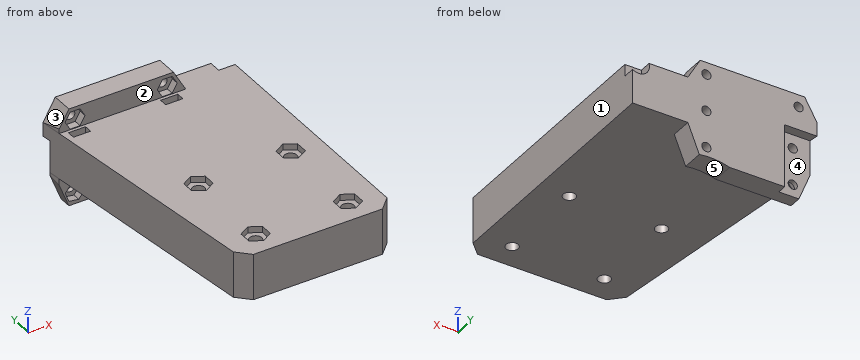
```python
from build123d import *

# Parameters (mm, degrees)
SKETCH1_W               = 50
SKETCH1_H               = 70
BOSS_EXTRUDE1_DEPTH     = 15
SKETCH3_R               = 2
CUT_EXTRUDE1_DEPTH      = 16
SKETCH4_W               = 50
SKETCH4_H               = 15
BOSS_EXTRUDE2_DEPTH     = 16
CHAMFER1_SIZE           = 4
BOSS_EXTRUDE3_DEPTH     = 15
SKETCH6_R               = 3.5
CUT_EXTRUDE2_DEPTH      = 4
SKETCH7_R               = 1.5
BOSS_EXTRUDE4_DEPTH     = 7
CUT_EXTRUDE3_DEPTH      = 8
CUT_EXTRUDE3_DEPTH_BACK = 26
SKETCH7_2_R             = 1.5
CUT_EXTRUDE4_DEPTH      = 20
SKETCH9_W               = 5.6
SKETCH9_H               = 2.6
CUT_EXTRUDE5_DEPTH      = 26
SKETCH10_W              = 10.5
SKETCH10_H              = 20.5
CUT_EXTRUDE6_DEPTH      = 3
CUT_EXTRUDE7_DEPTH      = 2.5
CUT_EXTRUDE8_DEPTH      = 2
SKETCH14_R              = 22
CUT_EXTRUDE9_DEPTH      = 87


with BuildPart() as part:
    # Sketch1 → Boss-Extrude1 (new body)
    with BuildSketch(Plane.XY):
        Rectangle(SKETCH1_W, SKETCH1_H)
    extrude(amount=BOSS_EXTRUDE1_DEPTH)

    # Sketch3 → Cut-Extrude1 (cut, through all)
    with BuildSketch(Plane.XY.offset(15)):
        with Locations((-15, 2.7)):
            Circle(SKETCH3_R)
        with Locations((15, 2.7)):
            Circle(SKETCH3_R)
        with Locations((-15, -26.7)):
            Circle(SKETCH3_R)
        with Locations((15, -26.7)):
            Circle(SKETCH3_R)
    extrude(amount=-CUT_EXTRUDE1_DEPTH, mode=Mode.SUBTRACT)

    # Sketch4 → Boss-Extrude2 (add)
    with BuildSketch(Plane(origin=(0, 35, 0), x_dir=(1, 0, 0), z_dir=(0, 1, 0))):
        with Locations((0, -7.5)):
            Rectangle(SKETCH4_W, SKETCH4_H)
    extrude(amount=BOSS_EXTRUDE2_DEPTH)

    # Chamfer1
    chamfer1_edges = [part.edges().sort_by_distance(p)[0] for p in [
        (25, -35, 7.5),
        (-25, -35, 7.5),
    ]]
    chamfer(chamfer1_edges, length=CHAMFER1_SIZE)

    # Sketch5 → Boss-Extrude3 (add)
    with BuildSketch(Plane.XY.offset(15)):
        Polygon((-25, 51), (-35, 51), (-25, -31), align=None)
    extrude(amount=-BOSS_EXTRUDE3_DEPTH)

    # Sketch6 → Cut-Extrude2 (cut)
    with BuildSketch(Plane(origin=(0, 51, 0), x_dir=(1, 0, 0), z_dir=(0, 1, 0))):
        with Locations((23, -14)):
            Circle(SKETCH6_R)
    extrude(amount=-CUT_EXTRUDE2_DEPTH, mode=Mode.SUBTRACT)

    # Sketch7 → Boss-Extrude4 (add)
    with BuildSketch(Plane(origin=(0, 51, 0), x_dir=(1, 0, 0), z_dir=(0, 1, 0))):
        with Locations((-29, -6)):
            Circle(SKETCH7_R)
        with Locations((1, -6)):
            Circle(SKETCH7_R)
        Polygon((-35, -15), (-31, -22), (3, -22), (7, -15), align=None)
        with Locations((-29, -18)):
            Circle(SKETCH7_R, mode=Mode.SUBTRACT)
        with Locations((1, -18)):
            Circle(SKETCH7_R, mode=Mode.SUBTRACT)
        Polygon((-35, 0), (-31, 10), (3, 10), (7, 0), align=None)
        with Locations((-29, 6)):
            Circle(SKETCH7_R, mode=Mode.SUBTRACT)
        with Locations((1, 6)):
            Circle(SKETCH7_R, mode=Mode.SUBTRACT)
    extrude(amount=-BOSS_EXTRUDE4_DEPTH)

    # Sketch8 → Cut-Extrude3 (cut, two sides)
    with BuildSketch(Plane.XY.offset(15)) as cut_extrude3_sk:
        Polygon((-35, 51), (-34.146341463, 44), (-33.909721647, 42.059717507), (-44.503182053, 47.14840404), (-41.913565843, 51), align=None)
    extrude(amount=CUT_EXTRUDE3_DEPTH, mode=Mode.SUBTRACT)
    extrude(cut_extrude3_sk.sketch, amount=-CUT_EXTRUDE3_DEPTH_BACK, mode=Mode.SUBTRACT)

    # Sketch7<2> → Cut-Extrude4 (cut)
    with BuildSketch(Plane(origin=(0, 51, 0), x_dir=(1, 0, 0), z_dir=(0, 1, 0))):
        with Locations((-29, -6)):
            Circle(SKETCH7_2_R)
        with Locations((1, -6)):
            Circle(SKETCH7_2_R)
    extrude(amount=-CUT_EXTRUDE4_DEPTH, mode=Mode.SUBTRACT)

    # Sketch9 → Cut-Extrude5 (cut, through all)
    with BuildSketch(Plane.XY.offset(15)):
        with Locations((-29, 41.7)):
            Rectangle(SKETCH9_W, SKETCH9_H)
        with Locations((1, 41.7)):
            Rectangle(SKETCH9_W, SKETCH9_H)
    extrude(amount=-CUT_EXTRUDE5_DEPTH, mode=Mode.SUBTRACT)

    # Sketch10 → Cut-Extrude6 (cut)
    with BuildSketch(Plane(origin=(0, 51, 0), x_dir=(1, 0, 0), z_dir=(0, 1, 0))):
        with Locations((-29.75, -0.25)):
            Rectangle(SKETCH10_W, SKETCH10_H)
    extrude(amount=-CUT_EXTRUDE6_DEPTH, mode=Mode.SUBTRACT)

    # Sketch11 → Cut-Extrude7 (cut)
    with BuildSketch(Plane.XZ.offset(-44)):
        Polygon((-30.999351715, -8.540851443), (-27.799233961, -9.001915098), (-25.799882246, -6.461063655), (-27.000648285, -3.459148557), (-30.200766039, -2.998084902), (-32.200117754, -5.538936345), align=None)
        Polygon((2.616580754, -8.8), (4.233161507, -6), (2.616580754, -3.2), (-0.616580754, -3.2), (-2.233161507, -6), (-0.616580754, -8.8), align=None)
        Polygon((-32.233129457, 17.985603874), (-30.604097318, 15.192829694), (-27.370967861, 15.207225819), (-25.766870543, 18.014396126), (-27.395902682, 20.807170306), (-30.629032139, 20.792774181), align=None)
        Polygon((2.629032139, 20.792774181), (-0.604097318, 20.807170306), (-2.233129457, 18.014396126), (-0.629032139, 15.207225819), (2.604097318, 15.192829694), (4.233129457, 17.985603874), align=None)
    extrude(amount=-CUT_EXTRUDE7_DEPTH, mode=Mode.SUBTRACT)

    # Sketch13 → Cut-Extrude8 (cut)
    with BuildSketch(Plane.XY.offset(15)):
        Polygon((11.5, 0.679274058), (15, -1.341451884), (18.5, 0.679274058), (18.5, 4.720725942), (15, 6.741451884), (11.5, 4.720725942), align=None)
        Polygon((-18.5, -28.720725942), (-15, -30.741451884), (-11.5, -28.720725942), (-11.5, -24.679274058), (-15, -22.658548116), (-18.5, -24.679274058), align=None)
        Polygon((18.5, -28.720725942), (18.5, -24.679274058), (15, -22.658548116), (11.5, -24.679274058), (11.5, -28.720725942), (15, -30.741451884), align=None)
        Polygon((-11.5, 4.720725942), (-15, 6.741451884), (-18.5, 4.720725942), (-18.5, 0.679274058), (-15, -1.341451884), (-11.5, 0.679274058), align=None)
    extrude(amount=-CUT_EXTRUDE8_DEPTH, mode=Mode.SUBTRACT)

    # Sketch14 → Cut-Extrude9 (cut, through all)
    with BuildSketch(Plane(origin=(0, 51, 0), x_dir=(1, 0, 0), z_dir=(0, 1, 0))):
        with Locations((0, 31)):
            Circle(SKETCH14_R)
    extrude(amount=-CUT_EXTRUDE9_DEPTH, mode=Mode.SUBTRACT)


solid = part.part
```
Verification items for the finished model (mm, model axes). Face numbers are marked on the shaded views. A direction names the side the tool comes from. Coordinates: 2 decimals unless noted, no trailing zeros. Write each loop counter-clockwise with the first axis right and the second up, starting at its lowest first coordinate (ties: lowest second). Pieces come first, ordered by that corner, then holes. Notation, with made-up numbers: M 49.5,-19.5 L 104.5,-19.5 A20 cw 104.5,-7.5 Z; hole C 2.5,-1.5 d10. An arc over 180 degrees is marked long. One line per item, written item: value.
Item 1: Section check B-B, the plane z = 6. State how many separate pieces and enclosed holes the cut face has, plus the area to 3 significant figures.
Check sheet entries:
separate pieces: 1
enclosed holes: 4
area: 4,490 mm^2
Item 2: Gauge pin test, flat ends, axial feed: pin 1 Ø10 at (y, z) = (0.5, 6.5) entering from -X; pin 2 Ø17.5 at (x, y) = (4, -12.5) entering from -Z; pin 3 Ø1.8 at (x, z) = (-29, -6) entering from +Y; pin 4 Ø4.5 at (x, z) = (-29, 4) entering from +Y. Record the tip position at first contact, or that the pin passes through.
Check sheet entries:
pin 1: stops at x = -29.45
pin 2: stops at z = 0
pin 3: passes through
pin 4: stops at y = 48
Item 3: Access from +Z, -Z, +X, -X, +Y, -Y to the whole of each face (thin tool, end or side, straight path). Record for the marked faces 1 and 2.
Check sheet entries:
face 1: +Z, -Z, +X, +Y, -Y
face 2: +Z, +X, -X, -Y
Item 4: Section check C-C, the plane y = 10. Record the boundary of the cut face in (x, z).
Check sheet entries:
outline: M -30,0 L 25,0 L 25,15 L -30,15 Z
Item 5: Scan lines: line 1 along Z through (x, y) = (1, 48.75); line 2 along Y through (x, z) = (15, 9); line 3 along X through (y, z) = (-25.5, 11). Record each from-to range of solid material in increasing order.
Check sheet entries:
line 1: z = -9.02 to -7.5, -4.5 to 4.5, 7.5 to 16.5, 19.5 to 22
line 2: y = -35 to -28.7, -24.7 to 0.7, 4.7 to 51
line 3: x = -25.67 to -16.6, -13.4 to 13.4, 16.6 to 25
Item 6: Mould release check, pull along X, two halves, no side actions. Record for the marked faces 3, 4 and 5: pulls with the +X half, pulls with the -X half, needs draft (parallel to the pull), parting line crosses it, or undercut.
Check sheet entries:
face 3: pulls with the -X half
face 4: needs draft
face 5: undercut
Item 7: Section check A-A, the plane x = 5.5. Record the boundary of the cut face in (y, z) (3 decimals), plus the area to 3 significant figures.
Check sheet entries:
outline: M -35,0 L 44,0 L 44,-3.75 L 51,-3.75 L 51,17.625 L 44,17.625 L 44,15 L -35,15 Z
area: 1,330 mm^2
